Could you check a few things on this model? Use its own coordinates, in mm. A direction names the side the tool comes from. Give positions to 0.01 mm unless a question says otherwise; leave off trailing zeros. Write each loop counter-clockwise with the first axis right and the second up, starting at its lowest first coordinate (ties: lowest second). Pieces come first, ordered by that corner, then holes. Notation, with made-up numbers: (69, 62.5) - (82, 62.5) arc R11 cw to (82, 67.5) - close; hole circle Ø1 at (23, -0.5). An arc over 180 degrees is marked (long way). Answer in a Markdown table with one row per item.
from build123d import *

# Parameters (mm, degrees)
BOSS_EXTRUDE2_START       = -4.5
SKETCH1_W                 = 30
SKETCH1_H                 = 3
BOSS_EXTRUDE2_DEPTH       = 5.5
SKETCH3_R                 = 44.5
SKETCH3_R_2               = 34.5
SKETCH3_R_3               = 1
BOSS_EXTRUDE3_DEPTH       = 2.5
CHAMFER1_SIZE             = 3
CHAMFER1_SIZE_2           = 0.803847577
FILLET1_R                 = 1.5
F_1_0MM_START             = -15
F_1_0MM_DOWEL_SLOT1_DEPTH = 30
CIRPATTERN1_COUNT         = 6
FILLET1_OF_CIRPATTERN1_R  = 1.5


# Read off the part's stored shape, not the designer's step: Ø1.0mm Dowel Slot1
with BuildPart() as part:
    # Sketch1 → Boss-Extrude2 (new body)
    with BuildSketch(Plane(origin=(0, 0, 0), x_dir=(1, 0, 0), z_dir=(0, 1, 0)).offset(BOSS_EXTRUDE2_START)):
        with Locations((0, -39.5)):
            Rectangle(SKETCH1_W, SKETCH1_H)
    boss_extrude2 = extrude(amount=BOSS_EXTRUDE2_DEPTH)

    # Sketch3 → Boss-Extrude3 (add)
    with BuildSketch(Plane(origin=(0, 0, 0), x_dir=(1, 0, 0), z_dir=(0, 1, 0))):
        with Locations(Location((0, 0, 0), (0, 0, 270))):
            Circle(SKETCH3_R)
        with Locations(Location((0, 0, 0), (0, 0, 270))):
            Circle(SKETCH3_R_2, mode=Mode.SUBTRACT)
        with Locations(Location((-20, 34.641016151, 0), (0, 0, 270))):
            Circle(SKETCH3_R_3, mode=Mode.SUBTRACT)
        with Locations(Location((20, 34.641016151, 0), (0, 0, 270))):
            Circle(SKETCH3_R_3, mode=Mode.SUBTRACT)
        with Locations(Location((40, 0, 0), (0, 0, 270))):
            Circle(SKETCH3_R_3, mode=Mode.SUBTRACT)
        with Locations(Location((20, -34.641016151, 0), (0, 0, 270))):
            Circle(SKETCH3_R_3, mode=Mode.SUBTRACT)
        with Locations(Location((-20, -34.641016151, 0), (0, 0, 270))):
            Circle(SKETCH3_R_3, mode=Mode.SUBTRACT)
        with Locations(Location((-40, 0, 0), (0, 0, 270))):
            Circle(SKETCH3_R_3, mode=Mode.SUBTRACT)
    extrude(amount=BOSS_EXTRUDE3_DEPTH)

    # Chamfer1
    # the kernel refuses this chamfer: 3, 0.803847577 mm, written as the material it takes off along each edge
    with BuildSketch(Plane(origin=(20, 2.5, 34.641016151), x_dir=(0, 0, 1), z_dir=(-1, 0, 0))) as chamfer1_piece_1:
        Polygon((1, -CHAMFER1_SIZE), (1 + CHAMFER1_SIZE_2, 0), (1, 0), align=None)
    revolve(axis=Axis((20, 2.5, 34.641016151), (0, 1, 0)), mode=Mode.SUBTRACT)
    with BuildSketch(Plane(origin=(40, 2.5, 0), x_dir=(0, 0, 1), z_dir=(-1, 0, 0))) as chamfer1_piece_2:
        Polygon((1, -CHAMFER1_SIZE), (1 + CHAMFER1_SIZE_2, 0), (1, 0), align=None)
    revolve(axis=Axis((40, 2.5, 0), (0, 1, 0)), mode=Mode.SUBTRACT)
    with BuildSketch(Plane(origin=(20, 2.5, -34.641016151), x_dir=(0, 0, 1), z_dir=(-1, 0, 0))) as chamfer1_piece_3:
        Polygon((1, -CHAMFER1_SIZE), (1 + CHAMFER1_SIZE_2, 0), (1, 0), align=None)
    revolve(axis=Axis((20, 2.5, -34.641016151), (0, 1, 0)), mode=Mode.SUBTRACT)
    with BuildSketch(Plane(origin=(-20, 2.5, -34.641016151), x_dir=(0, 0, 1), z_dir=(-1, 0, 0))) as chamfer1_piece_4:
        Polygon((1, -CHAMFER1_SIZE), (1 + CHAMFER1_SIZE_2, 0), (1, 0), align=None)
    revolve(axis=Axis((-20, 2.5, -34.641016151), (0, 1, 0)), mode=Mode.SUBTRACT)
    with BuildSketch(Plane(origin=(-40, 2.5, 0), x_dir=(0, 0, 1), z_dir=(-1, 0, 0))) as chamfer1_piece_5:
        Polygon((1, -CHAMFER1_SIZE), (1 + CHAMFER1_SIZE_2, 0), (1, 0), align=None)
    revolve(axis=Axis((-40, 2.5, 0), (0, 1, 0)), mode=Mode.SUBTRACT)
    with BuildSketch(Plane(origin=(-20, 2.5, 34.641016151), x_dir=(0, 0, 1), z_dir=(-1, 0, 0))) as chamfer1_piece_6:
        Polygon((1, -CHAMFER1_SIZE), (1 + CHAMFER1_SIZE_2, 0), (1, 0), align=None)
    revolve(axis=Axis((-20, 2.5, 34.641016151), (0, 1, 0)), mode=Mode.SUBTRACT)

    # Fillet1
    fillet1_edges = [part.edges().sort_by_distance(p)[0] for p in [
        (-15, -4.5, 39.5),
        (15, -4.5, 39.5),
    ]]
    fillet(fillet1_edges, radius=FILLET1_R)

    # Ø1.0mm Dowel Slot1 outline → Ø1.0mm Dowel Slot1 (cut)
    with BuildSketch(Plane.YZ.offset(F_1_0MM_START)):
        with BuildLine():
            ThreePointArc((-1.5, 38), (-1.866116524, 38.883883476), (-2.75, 39.25))
            Line((-2.75, 39.25), (-3.25, 39.25))
            ThreePointArc((-3.25, 39.25), (-4.133883476, 38.883883476), (-4.5, 38))
            Line((-4.5, 38), (-1.5, 38))
        make_face()
    f_1_0mm_dowel_slot1 = extrude(amount=F_1_0MM_DOWEL_SLOT1_DEPTH, mode=Mode.SUBTRACT)

    # CirPattern1: Boss-Extrude2, Ø1.0mm Dowel Slot1 ×6 about axis
    cirpattern1_axis = Axis((0, 0, 0), (0, 1, 0))
    add([boss_extrude2.rotate(cirpattern1_axis, i * 360 / CIRPATTERN1_COUNT) for i in range(1, CIRPATTERN1_COUNT)])
    add([f_1_0mm_dowel_slot1.rotate(cirpattern1_axis, i * 360 / CIRPATTERN1_COUNT) for i in range(1, CIRPATTERN1_COUNT)], mode=Mode.SUBTRACT)

    # Fillet1 of CirPattern1
    fillet1_of_cirpattern1_edges = [part.edges().sort_by_distance(p)[0] for p in [
        (26.708003449, -4.5, 32.740381057),
        (41.708003449, -4.5, 6.759618943),
        (41.708003449, -4.5, -6.759618943),
        (26.708003449, -4.5, -32.740381057),
        (15, -4.5, -39.5),
        (-15, -4.5, -39.5),
        (-26.708003449, -4.5, -32.740381057),
        (-41.708003449, -4.5, -6.759618943),
        (-41.708003449, -4.5, 6.759618943),
        (-26.708003449, -4.5, 32.740381057),
    ]]
    fillet(fillet1_of_cirpattern1_edges, radius=FILLET1_OF_CIRPATTERN1_R)


solid = part.part
1) On a 3-axis mill with a long thin cutter (end or side, diameter ignored), from which of +Z, -Z, +X, -X, +Y, -Y can I reach the whole of each face in a straight line? I mean faces 1 (the face through (42.015, -1.188, -6.937)), 2 (the face through (32.804, -0.76, 19.182)), 3 (the face through (0, -2, 41)). Say none if no direction works.
Check values:
| item | result |
|---|---|
| face 1 | +X, -Y |
| face 2 | -Y |
| face 3 | +Z, +X, -X, -Y |
2) Imagine slicing it at C-C (x = 20). List the corners of the cut face in (y, z) for me (3 decimals), then the cut area to 3 significant figures.
Check values:
| item | result |
|---|---|
| outline | (0, -39.752) - (2.5, -39.752) - (2.5, -36.445) - (0, -35.775) - close; (0, -33.507) - (2.5, -32.837) - (2.5, -28.111) - (0, -28.111) - close; (0, 28.111) - (2.5, 28.111) - (2.5, 32.837) - (0, 33.507) - close; (0, 35.775) - (2.5, 36.445) - (2.5, 39.752) - (0, 39.752) - close |
| area | 43.5 mm2 |
3) Imagine slicing it at B-B (z = 0). List the corners of the cut face in (x, y) for me.
Check values:
| item | result |
|---|---|
| outline | (-44.5, 0) - (-41.13, 0) - (-41.8, 2.5) - (-44.5, 2.5) - close; (-38.87, 0) - (-34.5, 0) - (-34.5, 2.5) - (-38.2, 2.5) - close; (34.5, 0) - (38.87, 0) - (38.2, 2.5) - (34.5, 2.5) - close; (41.13, 0) - (44.5, 0) - (44.5, 2.5) - (41.8, 2.5) - close |
4) Will these pins go through, and if not, where does the flat tip stop? P1, Ø2.5, axis at y = -2, z = 40, coming from the +X side; P2, Ø1.2, axis at x = -7.5, y = -0.5, coming from the -Z side; P3, Ø3, axis at x = -13.5, z = -28, coming from the +Y side; P4, Ø3.5, axis at y = -1, z = -39, coming from the -X side.
Check values:
| item | result |
|---|---|
| P1 | stops at x = 15 |
| P2 | stops at z = -43.92 |
| P3 | passes through |
| P4 | stops at x = -23.86 |
5) Imagine slicing it at A-A (x = 0). List the corners of the cut face in (y, z) for me.
Check values:
| item | result |
|---|---|
| outline | (-4.5, -41) - (0, -41) - (0, -44.5) - (2.5, -44.5) - (2.5, -34.5) - (0, -34.5) - (0, -38) - (-1.5, -38) arc R1.25 cw to (-2.75, -39.25) - (-3.25, -39.25) arc R1.25 cw to (-4.5, -38) - close; (-4.5, 38) arc R1.25 cw to (-3.25, 39.25) - (-2.75, 39.25) arc R1.25 cw to (-1.5, 38) - (0, 38) - (0, 34.5) - (2.5, 34.5) - (2.5, 44.5) - (0, 44.5) - (0, 41) - (-4.5, 41) - close |
6) We'd pull the mould along Y, two halves only. Please class faces 4 (the face through (-33.561, -1.856, -19.619)), 5 (the face through (0, -2, -41)), 6 (the face through (-27.29, -4.22, -32.35)): +Y half, -Y half, draft (parallel to the pull), parting line (faces both ways), or undercut.
Check values:
| item | result |
|---|---|
| face 4 | undercut |
| face 5 | draft |
| face 6 | -Y half |
7) If I drill on line 1 (Z direction, x = -7, y = -1); line 2 (X direction, y = 1.5, z = 0); line 3 (X direction, y = 2, z = 17), over which ranges is the centre line in solid material (lowest first)?
Check values:
| item | result |
|---|---|
| line 1 | z = -41 to -38, 38 to 41 |
| line 2 | x = -44.5 to -41.54, -38.46 to -34.5, 34.5 to 38.46, 41.54 to 44.5 |
| line 3 | x = -41.12 to -30.02, 30.02 to 41.12 |
